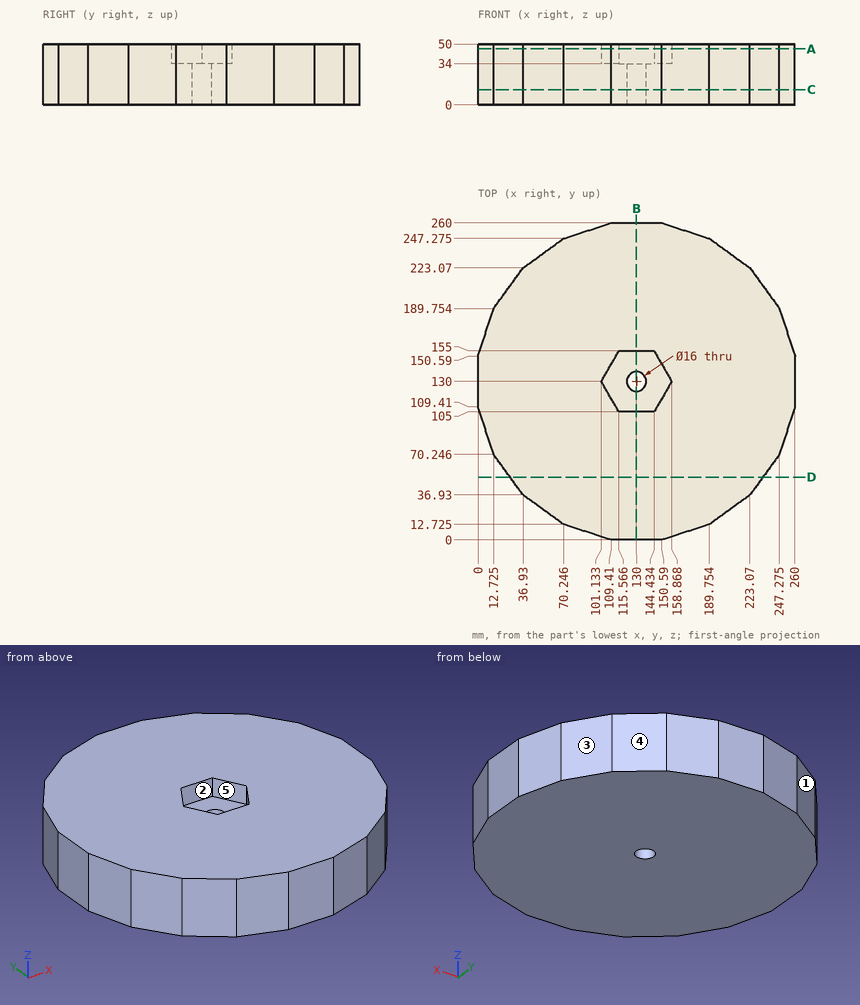
Here's the drawing with two shaded views (mm, measured from the low corner). I have some questions. A direction names the side the tool comes from. Round coordinates to 2 decimals unless told otherwise and drop trailing zeros. Order: outer loops, then holes, each group sorted by start corner. A loop starts at its lowest first (then second) coordinate and runs counter-clockwise, first axis right, second up. Notation, with made-up numbers: M 5.5,82 L 15.5,82 A15 cw 15.5,103 Z; hole C 86,-22.5 d10. An arc over 180 degrees is marked long. Use CSV: the item, a comma, the result in double quotes.
1) I want a section at A-A (z = 46). List the corners of the cut face in (x, y) for me (1 decimal), then the cut area to 3 significant figures.
Taken from the geometry:
outline,"M 0,109.4 L 12.7,70.2 L 36.9,36.9 L 70.2,12.7 L 109.4,0 L 150.6,0 L 189.8,12.7 L 223.1,36.9 L 247.3,70.2 L 260,109.4 L 260,150.6 L 247.3,189.8 L 223.1,223.1 L 189.8,247.3 L 150.6,260 L 109.4,260 L 70.2,247.3 L 36.9,223.1 L 12.7,189.8 L 0,150.6 Z; hole M 101.1,130 L 115.6,105 L 144.4,105 L 158.9,130 L 144.4,155 L 115.6,155 Z"
area,"51,400 mm^2"
2) I want a section at B-B (x = 130). List the corners of the cut face in (y, z) for me, then the cut area to 3 significant figures.
Taken from the geometry:
outline,"M 0,0 L 122,0 L 122,34 L 105,34 L 105,50 L 0,50 Z; M 138,0 L 260,0 L 260,50 L 155,50 L 155,34 L 138,34 Z"
area,"11,700 mm^2"
3) On a 3-axis mill with a long thin cutter (end or side, diameter ignored), from which of +Z, -Z, +X, -X, +Y, -Y can I reach the whole of each face in a straight line? I mean the marked faces 4 and 5. Say none if no direction works.
Taken from the geometry:
face 4,"+Z, -Z, +X, +Y"
face 5,"+Z"
4) I'm going to push flat-ended pins straight in: P1, Ø6, axis at x = 115.5, y = 116.5, coming from the +Z side; P2, Ø6, axis at x = 75.5, z = 18.5, coming from the +Y side; P3, Ø10, axis at y = 57.5, z = 41.5, coming from the +X side. Where does each tip first touch, or does it pass through?
Taken from the geometry:
P1,"z = 34"
P2,"y = 249.96"
P3,"x = 241.65"
5) I want a section at D-D (y = 51.5). List the corners of the cut face in (x, z) for me (1 decimal).
Taken from the geometry:
outline,"M 26.3,0 L 233.7,0 L 233.7,50 L 26.3,50 Z"
6) If we mould it in two halves opening along X, with no side actions, what happens to the marked faces 1, 2 and 3? For each: pulls with the +X half, pulls with the -X half, needs draft (parallel to the pull), parting line crosses it, or undercut.
Taken from the geometry:
face 1,"pulls with the -X half"
face 2,"undercut"
face 3,"pulls with the +X half"
7) I need wall thicknesses on line 1 along Y through (x, z) = (130, 24); line 2 along Y through (x, z) = (126.5, 17) (1 decimal); line 3 along Z through (x, y) = (145, 145). Which ranges of each line are inside material? Lowest first, please. Write a range as [from, to].
Taken from the geometry:
line 1,"[0, 122], [138, 260]"
line 2,"[0, 122.8], [137.2, 260]"
line 3,"[0, 34]"
8) I want a section at C-C (z = 12.5). List the corners of the cut face in (x, y) for me (1 decimal), then the cut area to 3 significant figures.
Taken from the geometry:
outline,"M 0,109.4 L 12.7,70.2 L 36.9,36.9 L 70.2,12.7 L 109.4,0 L 150.6,0 L 189.8,12.7 L 223.1,36.9 L 247.3,70.2 L 260,109.4 L 260,150.6 L 247.3,189.8 L 223.1,223.1 L 189.8,247.3 L 150.6,260 L 109.4,260 L 70.2,247.3 L 36.9,223.1 L 12.7,189.8 L 0,150.6 Z; hole C 130,130 d16"
area,"53,300 mm^2"
